Geometry check sheet. Reference: the model listing, model coordinates, mm. A direction names the side the tool comes from. Coordinates: 2 decimals unless noted, no trailing zeros. Write each loop counter-clockwise with the first axis right and the second up, starting at its lowest first coordinate (ties: lowest second). Pieces come first, ordered by that corner, then holes.
from build123d import *

# Parameters (mm, degrees)
SKETCH1_R           = 10.16
BOSS_EXTRUDE1_DEPTH = 2.54
SKETCH2_R           = 3.81
BOSS_EXTRUDE2_DEPTH = 30.48
BOSS_EXTRUDE3_DEPTH = 3.81
FILLET1_R           = 1.27


with BuildPart() as part:
    # Sketch1 → Boss-Extrude1 (new body)
    with BuildSketch(Plane(origin=(0, 0, 0), x_dir=(1, 0, 0), z_dir=(0, 1, 0))):
        Circle(SKETCH1_R)
    extrude(amount=BOSS_EXTRUDE1_DEPTH)

    # Sketch2 → Boss-Extrude2 (add)
    with BuildSketch(Plane(origin=(0, 2.54, 0), x_dir=(1, 0, 0), z_dir=(0, 1, 0))):
        Circle(SKETCH2_R)
    extrude(amount=BOSS_EXTRUDE2_DEPTH)

    # Sketch3 → Boss-Extrude3 (add)
    with BuildSketch(Plane(origin=(0, 33.02, 0), x_dir=(1, 0, 0), z_dir=(0, 1, 0))):
        Polygon((2.104204897, 5.08), (-2.104204897, 5.08), (-5.08, 2.104204897), (-5.08, -2.104204897), (-2.104204897, -5.08), (2.104204897, -5.08), (5.08, -2.104204897), (5.08, 2.104204897), align=None)
    extrude(amount=BOSS_EXTRUDE3_DEPTH)

    # Fillet1
    fillet1_edges = [part.edges().sort_by_distance(p)[0] for p in [
        (5.08, 34.925, -2.104204897),
        (2.104204897, 34.925, -5.08),
        (-2.104204897, 34.925, -5.08),
        (-5.08, 34.925, -2.104204897),
        (-5.08, 34.925, 2.104204897),
        (-2.104204897, 34.925, 5.08),
        (2.104204897, 34.925, 5.08),
        (5.08, 34.925, 2.104204897),
        (3.592102448, 36.83, -3.592102448),
        (0, 36.83, -5.08),
        (-3.592102448, 36.83, -3.592102448),
        (-5.08, 36.83, 0),
        (-3.592102448, 36.83, 3.592102448),
        (0, 36.83, 5.08),
        (3.592102448, 36.83, 3.592102448),
        (5.08, 36.83, 0),
    ]]
    fillet(fillet1_edges, radius=FILLET1_R)


solid = part.part
1. Sectioned sample at D-D, the plane x = 8. Record the boundary of the cut face in (y, z).
Computed values:
outline: (0, -6.26) - (2.54, -6.26) - (2.54, 6.26) - (0, 6.26) - close
2. Sectioned sample at C-C, the plane y = 18. Record the boundary of the cut face in (x, z).
Computed values:
outline: circle Ø7.62 at (0, 0)
3. Gauge pin test, flat ends, axial feed: pin 1 Ø11 at (x, z) = (-1.5, 2) entering from -Y; pin 2 Ø3 at (y, z) = (31.5, -8) entering from +X; pin 3 Ø8 at (y, z) = (31.5, 3) entering from +X; pin 4 Ø2 at (x, y) = (0.5, 34) entering from +Z. Record the tip position at first contact, or that the pin passes through.
Computed values:
pin 1: stops at y = 0
pin 2: passes through
pin 3: stops at x = 5.08
pin 4: stops at z = 5.08
4. Thickness scan on line 1 along Y through (x, z) = (5.75, 1.25); line 2 along Z through (x, y) = (0, 18); line 3 along X through (y, z) = (17, 2). Record the ranges inside material, lowest first.
Computed values:
line 1: y = 0 to 2.54
line 2: z = -3.81 to 3.81
line 3: x = -3.24 to 3.24
5. Access from +Z, -Z, +X, -X, +Y, -Y to the whole of each face (thin tool, end or side, straight path). Record for faces 1 (the flat face through (3.608, 34.272, -3.576)), 2 (the cylindrical face through (-2.07, 34.31, 4.98)), 3 (the cylindrical face through (-2.058, 34.308, -4.986)), 4 (the cylindrical face through (2.07, 34.31, 4.98)), 5 (the flat face through (0, 34, 5.08)).
Computed values:
face 1: -Z, +X, +Y
face 2: +Z, -X, +Y
face 3: -Z, -X, +Y
face 4: +Z, +X, +Y
face 5: +Z, +X, -X, +Y
6. Sectioned sample at A-A, the plane z = 1. Record the boundary of the cut face in (x, y), and give its area (3 significant figures).
Computed values:
outline: (-10.11, 0) - (10.11, 0) - (10.11, 2.54) - (3.68, 2.54) - (3.68, 33.02) - (5.08, 33.02) - (5.08, 35.56) arc R1.27 ccw to (3.81, 36.83) - (-3.81, 36.83) arc R1.27 ccw to (-5.08, 35.56) - (-5.08, 33.02) - (-3.68, 33.02) - (-3.68, 2.54) - (-10.11, 2.54) - close
area: 313 mm2
7. Sectioned sample at B-B, the plane x = 0. Record the boundary of the cut face in (y, z).
Computed values:
outline: (0, -10.16) - (2.54, -10.16) - (2.54, -3.81) - (33.02, -3.81) - (33.02, -5.08) - (35.56, -5.08) arc R1.27 ccw to (36.83, -3.81) - (36.83, 3.81) arc R1.27 ccw to (35.56, 5.08) - (33.02, 5.08) - (33.02, 3.81) - (2.54, 3.81) - (2.54, 10.16) - (0, 10.16) - close
